Autodesk Inventor part; units mm, degrees
ref_plane "Work Plane1" through (8.8407, 0, -5.778) normal (0, 0, -1) x (-1, 0, 0)
ref_plane "YZ Plane" through (0, 0, 0) normal (1, 0, 0) x (0, 1, 0)
ref_plane "XZ Plane" through (0, 0, 0) normal (0, 1, 0) x (-1, 0, 0)
sketch "Sketch2" plane through (0, 0, 0) normal (0, 1, 0) x (-1, 0, 0)
  line L0 (11.1593, 9.222) -> (-8.8407, 9.222)
  line L1 (-8.8407, 9.222) -> (-8.8407, -20.778)
  line L2 (-8.8407, -20.778) -> (11.1593, -20.778)
  line L3 (11.1593, -20.778) -> (11.1593, 9.222)
  point P0 (0, 0)
  dimension "d23" = 30
  dimension "d24" = 20
extrude "Extrusion2" add sketch "Sketch2" along normal blind 3
sketch "Sketch3" plane through (0, 3, 0) normal (0, 1, 0) x (1, 0, 0)
  line L0 (8.8407, -9.222) -> (8.8407, 20.778)
  line L1 (8.8407, 20.778) -> (-11.1593, 20.778)
  line L2 (-11.1593, 20.778) -> (-11.1593, -9.222)
  line L3 (-11.1593, -9.222) -> (8.8407, -9.222)
  line L4 (8.8407, -9.222) -> (8.8407, 20.778)
  line L5 (8.8407, 5.778) -> (-11.1593, 5.778)
  line L6 (-11.1593, 20.778) -> (-11.1593, -9.222)
  line L7 (8.8407, -7.222) -> (-11.1593, -7.222)
  line L8 (3.8407, -7.222) -> (-6.1593, -7.222)
  line L9 (-6.1593, -7.222) -> (-6.1593, 5.778)
  line L10 (-6.1593, 5.778) -> (3.8407, 5.778)
  line L11 (3.8407, 5.778) -> (3.8407, -7.222)
  line L12 (8.8407, 20.778) -> (8.8407, -9.222)
  line L13 (-11.1593, -9.222) -> (-11.1593, 20.778)
  line L14 (-11.1593, 20.778) -> (8.8407, 20.778)
  line L15 (8.8407, 20.778) -> (8.8407, -9.222)
  line L16 (-11.1593, -9.222) -> (-11.1593, 20.778)
  line L17 (8.8407, 18.778) -> (-11.1593, 18.778)
  line L18 (3.8407, 18.778) -> (-6.1593, 18.778)
  line L19 (-6.1593, 18.778) -> (-6.1593, 5.778)
  line L20 (3.8407, 5.778) -> (3.8407, 18.778)
  point P0 (0, 0)
  point P1 (8.8407, 18.778)
  point P2 (-11.1593, 18.778)
  point P3 (-6.1593, 18.778)
  point P4 (-6.1593, -7.222)
  dimension "d27" = 2
  dimension "d28" = 10
  dimension "d29" = 5
  dimension "d53" = 20
extrude "Extrusion3" add sketch "Sketch3" along normal blind 3 contours L3 L2 L7 L0 | L7 L9 L5 L11 | L17 L2 L1 L0 | L5 L19 L17 L20
sketch "Sketch4" plane through (0, 6, 0) normal (0, 1, 0) x (1, 0, 0)
  line L0 (8.8407, -7.222) -> (3.8407, -7.222)
  line L1 (8.8407, -9.222) -> (8.8407, -7.222)
  line L2 (8.8407, -7.222) -> (3.8407, -7.222)
  line L3 (3.8407, -7.222) -> (3.8407, 18.778)
  line L4 (3.8407, 18.778) -> (8.8407, 18.778)
  line L5 (8.8407, 18.778) -> (8.8407, 20.778)
  line L6 (8.8407, 20.778) -> (-11.1593, 20.778)
  line L7 (-11.1593, 20.778) -> (-11.1593, 18.778)
  line L8 (-11.1593, 18.778) -> (-6.1593, 18.778)
  line L9 (-6.1593, 18.778) -> (-6.1593, -7.222)
  line L10 (-6.1593, -7.222) -> (-11.1593, -7.222)
  line L11 (-11.1593, -7.222) -> (-11.1593, -9.222)
  line L12 (-11.1593, -9.222) -> (8.8407, -9.222)
  line L13 (8.8407, -7.222) -> (-11.1593, -7.222)
  line L14 (8.8407, -9.222) -> (8.8407, 20.778)
  line L15 (-11.1593, 18.778) -> (-11.1593, -7.222)
  line L16 (-11.1593, 18.778) -> (8.8407, 18.778)
  point P0 (0, 0)
extrude "Extrusion4" add sketch "Sketch4" along normal blind 5 contours L1 L12 L11 L10 L13 L0 | L4 L16 L8 L7 L6 L5
ref_plane "Work Plane1" through (8.8407, 0, -5.778) normal (0, 0, -1) x (-1, 0, 0)
chamfer "Chamfer1" distance 1 angle 80 2 edges at (8.8407, 11, 8.222) (-11.1593, 11, 8.222) measured on face at (2.174, 11, 8.5554)
chamfer "Chamfer2" distance 1 angle 80 2 edges at (8.8407, 11, -19.778) (-11.1593, 11, -19.778) measured on face at (2.174, 11, -19.4446)
sketch "Sketch5" plane through (0, 6, 0) normal (0, 1, 0) x (1, 0, 0)
  line L0 (-6.1593, -7.222) -> (3.8407, -7.222)
  line L1 (3.8407, -7.222) -> (3.8407, 18.778)
  line L2 (3.8407, 18.778) -> (-6.1593, 18.778)
  line L3 (-6.1593, 18.778) -> (-6.1593, -7.222)
  line L4 (3.8407, -5.222) -> (-6.1593, -5.222)
  line L5 (-6.1593, 18.778) -> (-6.1593, -7.222)
  line L6 (-15.1593, 5.778) -> (12.8407, 5.778)
  line L7 (3.8407, 16.778) -> (-6.1593, 16.778)
  point P0 (0, 0)
  point P1 (3.8407, 16.778)
  point P2 (-6.1593, 16.778)
  dimension "d40" = 11
  dimension "d54" = 26
extrude "Extrusion5" add sketch "Sketch5" along normal blind 4 contours L3 L6 L1 L4 | L3 L7 L1 L6
sketch "Sketch6" plane through (0, 10, 0) normal (0, 1, 0) x (1, 0, 0)
  line L0 (-6.1593, -7.222) -> (-6.1593, 18.778)
  line L1 (3.8407, 18.778) -> (3.8407, -7.222)
  line L2 (3.8407, -5.222) -> (3.8407, -2.0792)
  line L3 (3.8407, -2.0792) -> (-6.1593, -2.0792)
  line L4 (-6.1593, -2.0792) -> (-6.1593, -5.222)
  line L5 (3.8407, 16.778) -> (-6.1593, 16.778)
  line L6 (-6.1593, -5.222) -> (3.8407, -5.222)
  line L7 (-6.1593, 5.778) -> (3.8407, 5.778)
  line L8 (3.8407, 13.6351) -> (-6.1593, 13.6351)
  point P0 (0, 0)
  point P1 (-6.1593, -2.0792)
  point P2 (-6.1593, 13.6351)
  point P3 (3.8407, 13.6351)
  dimension "d43" = 22
  dimension "d44" = 3.1429
extrude "Extrusion6" add sketch "Sketch6" along normal blind 12 contours L0 L3 L1 L6 | L0 L5 L1 L8
fillet "Fillet1" radius 5 4 edges at (3.8407, 22, 3.6506) (-6.1593, 22, 3.6506) (-6.1593, 22, -15.2065) (3.8407, 22, -15.2065)
fillet "Fillet2" radius 5 2 edges at (-11.1593, 0, -5.778) (8.8407, 0, -5.778)
fillet "Fillet3" radius 5 2 edges at (-1.1593, 10, -13.6351) (-1.1593, 10, 2.0792)
sketch "Sketch9" plane through (-10.1593, 11, 9.222) normal (0, 0, 1) x (1, 0, 0)
  line L0 (0, 0) -> (18, 0)
  line L1 (4, -5) -> (4, 6)
  line L2 (14, -5) -> (14, 6)
  line L3 (0, 0) -> (18, 0)
  line L4 (4, 0) -> (14, 0)
  line L5 (14, 0) -> (14, -7)
  line L6 (14, -7) -> (4, -7)
  line L7 (4, -7) -> (4, 0)
  line L8 (4, -1) -> (14, -1)
  point P0 (10.1593, -11)
  point P1 (14, -1)
  point P2 (4, -1)
  dimension "d58" = 6
  dimension "d59" = 1
  dimension "d62" = 10
extrude "Extrusion8" add sketch "Sketch9" along normal blind 1 contours L8 L2 L5 L6 L7 L1
sketch "Sketch10" plane through (-6.1593, 6, 5.222) normal (0, 0, 1) x (1, 0, 0)
  circle A0 centre (5, 11) radius 2
  arc A1 (10, 11) -> (0, 11) centre (5, 11) ccw
  point P0 (6.1593, -6)
  dimension "d63" = 4
extrude "Extrusion9" cut sketch "Sketch10" against normal through all
chamfer "Chamfer3" distance 2 angle 45 10 edges at (-1.1593, 0, 9.222) (7.3762, 1.4645, 9.222) (8.8407, 5.1644, 9.222) (-9.6948, 1.4645, 9.222) (-11.1593, 5.1644, 9.222) (-1.1593, 0, -20.778) (-9.6948, 1.4645, -20.778) (-11.1593, 5.1644, -20.778) (7.3762, 1.4645, -20.778) (8.8407, 5.1644, -20.778)
chamfer "Chamfer4" distance 4 angle 45 2 edges at (-6.1593, 3, -5.778) (3.8407, 3, -5.778)
equation "\"d27\" = 0.1 * d53"
equation "\"d28\" = 0.5 * d53"
equation "\"d29\" = 0.25 * d53"
equation "\"d44\" = 0.142857 * d43"
properties part number "uchytka_spojky_medzi_velkym_strednym"
Work out the finished part from the listing and answer in its coordinate system (mm). A direction names the side the tool comes from. Give positions to 0.01 mm unless a question says otherwise; leave off trailing zeros. Loops run counter-clockwise (first coordinate to the right, second up) from the corner with the lowest first, then second, coordinate; pieces in that order, holes last. Notation, with made-up numbers: (83, 49.25) -> (116, 49.25) arc R23 cw to (116, 70.25) -> close; hole circle Ø6 at (82, 32). An arc over 180 degrees is marked (long way). Use a Markdown table: item, result. Add a question column.
1. Determine the mould class of faces 4 (the flat face through (-9.95, 7.96, 8.43)), 5 (the cylindrical face through (-1.229, 11.504, -12.209)), 6 (the flat face through (8.237, 8.755, -19.16)) for opening direction Z: released by +Z, released by -Z, zero draft, split by the parting line, or undercut.
2. For faces 1 (the flat face through (-1, 4, 10)), 2 (the flat face through (3.841, 7, 10)), 3 (the flat face through (-1, 14, 5.222)), determine the directions among +Z, -Z, +X, -X, +Y, -Y from which every point of the face is accessible in a straight line to the end or side of a thin tool.
3. Flat-ended cylindrical pins translate along their axes: pin 1 Ø2 at (x, y) = (0, 18) entering from +Z; pin 2 Ø4 at (y, z) = (7, -7) entering from -X; pin 3 Ø0.6 at (x, z) = (-5.5, 8) entering from +Y. Find the tip coordinate at first contact, or state that the pin passes through.
4. Section C-C on x = -5.5 is taken. Determine the outline of the cut face in (y, z).
5. Section A-A on z = -17.5 is taken. Determine the outline of the cut face in (x, y), and give its area (3 significant figures).
6. Find the intervals of material crossed by probe 1 along Z at (x, y) = (1, 8); probe 2 along Z at (x, y) = (2.25, 16.5); probe 3 along X at (y, z) = (17, 4.55), in increasing order.
7. Section B-B on y = 9 is taken. Determine the outline of the cut face in (x, z), and give its area (3 significant figures).
Results below:
| question | item | result |
|---|---|---|
| 1 | face 4 | released by +Z |
| 1 | face 5 | undercut |
| 1 | face 6 | zero draft |
| 2 | face 1 | +Z, +X, -X, -Y |
| 2 | face 2 | +Z, +X, +Y, -Y |
| 2 | face 3 | +X, -X, +Y |
| 3 | pin 1 | stops at z = 5.22 |
| 3 | pin 2 | stops at x = -8.16 |
| 3 | pin 3 | stops at y = 11 |
| 4 | outline | (0, -18.78) -> (2, -20.78) -> (11, -20.78) -> (11, -18.78) -> (6, -18.78) -> (6, -16.78) -> (19.48, -16.78) -> (19.48, -13.64) -> (15, -13.64) arc R5 cw to (10, -8.64) -> (10, -2.92) arc R5 cw to (15, 2.08) -> (19.48, 2.08) -> (19.48, 5.22) -> (6, 5.22) -> (6, 7.22) -> (11, 7.22) -> (11, 9.22) -> (10, 9.22) -> (10, 10.22) -> (4, 10.22) -> (4, 9.22) -> (2, 9.22) -> (0, 7.22) -> close |
| 5 | outline | (-10.74, 3) arc R5 ccw to (-6.16, 0) -> (3.84, 0) arc R5 ccw to (8.42, 3) -> (7.84, 3) -> (4.84, 6) -> (-7.16, 6) -> (-10.16, 3) -> close |
| 5 | area | 94.8 mm^2 |
| 6 | probe 1 | z = -20.78 to -18.78, -16.78 to 5.22, 7.22 to 10.22 |
| 6 | probe 2 | z = -16.78 to -13.64, 2.08 to 5.22 |
| 6 | probe 3 | x = -6.16 to -3.16, 0.84 to 3.84 |
| 7 | outline | (-10.51, -19.43) -> (-9.16, -20.78) -> (6.84, -20.78) -> (8.19, -19.43) -> (8.19, -18.78) -> (-10.51, -18.78) -> close; (-10.51, 7.22) -> (8.19, 7.22) -> (8.19, 7.87) -> (6.84, 9.22) -> (3.84, 9.22) -> (3.84, 10.22) -> (-6.16, 10.22) -> (-6.16, 9.22) -> (-9.16, 9.22) -> (-10.51, 7.87) -> close; (-6.16, -16.78) -> (3.84, -16.78) -> (3.84, 5.22) -> (-6.16, 5.22) -> close |
| 7 | area | 301 mm^2 |
